Solid Edge part; units mm, degrees
sketch "Sketch1" plane through (-29, 0, 0) normal (1, 0, 0) x (0, 1, 0)
  circle A0 centre (-9.5, 0) radius 2.2
  line L0 (15, -10.5) -> (-15, -10.5)
  line L1 (-15, -10.5) -> (-15, 10.5)
  line L2 (-15, 10.5) -> (15, 10.5)
  line L3 (15, 10.5) -> (15, -10.5)
  circle A1 centre (9.5, 0) radius 2.2
  dimension "D1" = 15
  dimension "D2" = 15
extrude "ExtrudedProtrusion_1" add sketch "Sketch1" against normal blind 18
sketch "Sketch2" plane through (-36.5, 0, 10.5) normal (0, 0, 1) x (0, -1, 0)
  circle A0 centre (0, 7.5) radius 4
extrude "Cutout1" cut sketch "Sketch2" against normal through all
Can you work these out from the model? Positions are in its coordinate system, mm. Round coordinates to 2 decimals unless told otherwise and drop trailing zeros. Loops run counter-clockwise (first coordinate to the right, second up) from the corner with the lowest first, then second, coordinate; pieces in that order, holes last. Notation, with made-up numbers: (3, -2.5) - (40, -2.5) arc R23 ccw to (40, 13.5) - close; hole circle Ø9 at (15, 17.5). An arc over 180 degrees is marked (long way). Write item = value, one per line. Start each with the question number.
(1) If we section it at C-C (x = -36.75): Please give me the cut outline in (y, z), and give its area (3 significant figures).
(2) If we section it at B-B (x = -32.5): Please give me the cut outline in (y, z), and give its area (3 significant figures).
(3) If we mould it in two halves opening along Y, with no side actions, what happens to faces 1 (the face through (-37.874, -11.698, 0.097)), 2 (the face through (-38, 15, 0)), 3 (the face through (-33, 0, 0)), 4 (the face through (-47, 0, 0))? For each: released by +Y, released by -Y, zero draft, split by the parting line, or undercut.
(4) If I drill on probe 1 along Z at (x, y) = (-36.75, -9.5); probe 2 along Y at (x, z) = (-43.25, -0.5); probe 3 along Y at (x, z) = (-39, 1.5), over which ranges is the centre line in solid material (lowest first)? Write a range as [from, to].
(5) For P1, Ø5, axis at y = -0.5, z = 6, coming from the +X side; P2, Ø7, axis at y = 9.5, z = 0, coming from the -X side, each with a flat end and sliding along its axis, tell me the tip position at first contact or that it passes through.
(6) If we section it at D-D (z = 3.25): Please give me the cut outline in (x, y), and give its area (3 significant figures).
(7) If we section it at A-A (y = -9.5): Please give me the cut outline in (x, z).
Ans:
q1.outline = (-15, -10.5) - (15, -10.5) - (15, 10.5) - (-15, 10.5) - close; hole circle Ø4.4 at (-9.5, 0); hole circle Ø4.4 at (9.5, 0)
q1.area = 600 mm²
q2.outline = (-15, -10.5) - (-1.94, -10.5) - (-1.94, 10.5) - (-15, 10.5) - close; (1.94, -10.5) - (15, -10.5) - (15, 10.5) - (1.94, 10.5) - close; hole circle Ø4.4 at (-9.5, 0); hole circle Ø4.4 at (9.5, 0)
q2.area = 518 mm²
q3.face_1 = undercut
q3.face_2 = released by +Y
q3.face_3 = undercut
q3.face_4 = zero draft
q4.probe_1 = [-10.5, -2.2], [2.2, 10.5]
q4.probe_2 = [-15, -11.64], [-7.36, 7.36], [11.64, 15]
q4.probe_3 = [-15, -11.11], [-7.89, 7.89], [11.11, 15]
q5.P1 = -31.65
q5.P2 = -47
q6.outline = (-47, -15) - (-29, -15) - (-29, -4) arc R4 cw to (-29, 4) - (-29, 15) - (-47, 15) - close
q6.area = 515 mm²
q7.outline = (-47, -10.5) - (-29, -10.5) - (-29, -2.2) - (-47, -2.2) - close; (-47, 2.2) - (-29, 2.2) - (-29, 10.5) - (-47, 10.5) - close
